Check sheet for the drawn part. Datum: minimum x, y, z corner. Units: mm. A direction names the side the tool comes from. Round coordinates to 2 decimals unless told otherwise and drop trailing zeros. Order: outer loops, then holes, each group sorted by start corner. A loop starts at its lowest first (then second) coordinate and runs counter-clockwise, first axis right, second up. Notation, with made-up numbers: (-4, 8) -> (0, 8) arc R5 cw to (0, 15) -> close; hole circle Ø5 at (72.25, 19.25). An arc over 180 degrees is marked (long way). Write item = value, one per line. Start each with the question number.
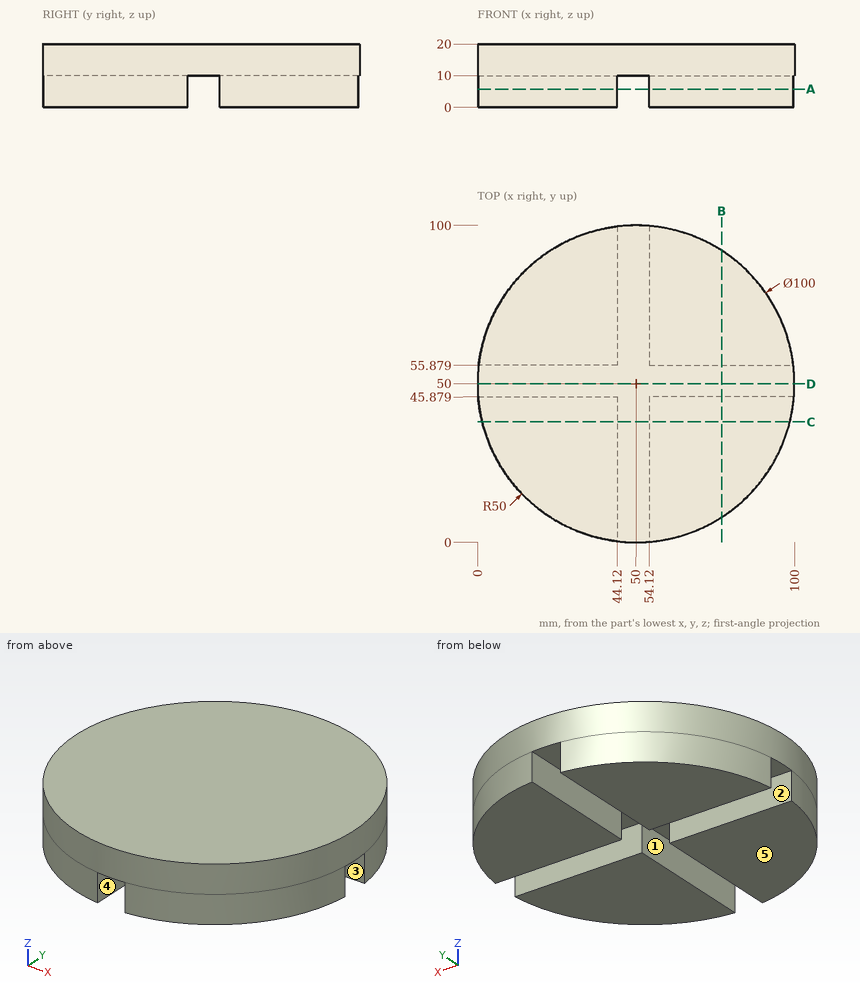
(1) Set-up check for the marked faces 3, 4 and 5: record each of +Z, -Z, +X, -X, +Y, -Y from which the full face is reachable in a straight line by a thin tool's end or side.
(2) Cross-section at C-C (y = 38). Enter the section's corners in (x, z).
(3) Scan lines: line 1 along X through (y, z) = (46, 19); line 2 along X through (y, z) = (13, 8.5); line 3 along Z through (x, y) = (47.5, 40). Record each from-to range of solid material in increasing order. Write a range as from..to.
(4) Draft check along X on the marked faces 1 and 2. Enter one of: +X half, -X half, draft (parallel to the pull), parting line (faces both ways), or undercut.
(5) Cross-section at B-B (x = 77). Enter the section's corners in (y, z).
(6) Cross-section at D-D (y = 50). Enter the section's corners in (x, z), and give its area (3 significant figures).
(7) Cross-section at A-A (z = 5.75). Enter the section's corners in (x, y).
(8) Depth check by flat-ended pin: pin 1 (12 mm diameter, centred on x = 23.5, z = 12, fed in from -Y) (1 decimal); pin 2 (8 mm diameter, centred on y = 20.5, z = 2.5, fed in from +X); pin 3 (1 mm diameter, centred on x = 34, z = 16.5, fed in from -Y). Enter the tip coordinate at first touch or a pass-through.
Outcome:
q1.face_3 = -Z, +X, -X
q1.face_4 = -Z, +Y, -Y
q1.face_5 = -Z, +X, -X, +Y, -Y
q2.outline = (1.46, 0) -> (44.12, 0) -> (44.12, 10) -> (54.12, 10) -> (54.12, 0) -> (98.54, 0) -> (98.54, 20) -> (1.46, 20) -> close
q3.line_1 = 0.16..99.84
q3.line_2 = 16.37..44.12, 54.12..83.63
q3.line_3 = 10..20
q4.face_1 = undercut
q4.face_2 = draft
q5.outline = (7.92, 0) -> (45.88, 0) -> (45.88, 10) -> (55.88, 10) -> (55.88, 0) -> (92.08, 0) -> (92.08, 20) -> (7.92, 20) -> close
q6.outline = (0, 10) -> (100, 10) -> (100, 20) -> (0, 20) -> close
q6.area = 1,000 mm^2
q7.outline = (0.17, 45.88) arc R50 ccw to (44.12, 0.35) -> (44.12, 45.88) -> close; (0.35, 55.88) -> (44.12, 55.88) -> (44.12, 99.65) arc R50 ccw to start; (54.12, 0.17) arc R50 ccw to (99.83, 45.88) -> (54.12, 45.88) -> close; (54.12, 55.88) -> (99.65, 55.88) arc R50 ccw to (54.12, 99.83) -> close
q8.pin_1 = 4.4
q8.pin_2 = 93.01
q8.pin_3 = 2.46
